from build123d import *

# Parameters (mm, degrees)
SKETCH_1_R                       = 10
EXTRUDE_1_DEPTH                  = 50
SKETCH_2_R                       = 10
EXTRUDE_2_DEPTH                  = 50
SKETCH_3_OUTSIDE_W               = 50.566
SKETCH_3_OUTSIDE_H               = 130.566
SKETCH_3_OUTSIDE_R               = 3
CUT_EXTRUDE_1_DEPTH              = 20
FILLET_2_R                       = 4
PATTERN_CIRCULAR_1_COUNT         = 4
FILLET_2_OF_PATTERN_CIRCULAR_1_R = 4


with BuildPart() as part:
    # Sketch 1 → Extrude 1 (new, symmetric)
    with BuildSketch(Plane(origin=(0, 0, 0), x_dir=(1, 0, 0), z_dir=(0, 1, 0))):
        with Locations(Location((0, 0, 0), (0, 0, 90))):
            Circle(SKETCH_1_R)
    extrude(amount=EXTRUDE_1_DEPTH, both=True)

    # Sketch 2 → Extrude 2 (add, symmetric)
    with BuildSketch(Plane(origin=(0, 0, 0), x_dir=(0, 0, -1), z_dir=(1, 0, 0))):
        Circle(SKETCH_2_R)
    extrude(amount=EXTRUDE_2_DEPTH, both=True)

    # Sketch 3 outside → Cut-Extrude 1 (cut)
    with BuildSketch(Plane.ZY.offset(50)):
        Rectangle(SKETCH_3_OUTSIDE_W, SKETCH_3_OUTSIDE_H)
        Circle(SKETCH_3_OUTSIDE_R, mode=Mode.SUBTRACT)
    cut_extrude_1 = extrude(amount=-CUT_EXTRUDE_1_DEPTH, mode=Mode.SUBTRACT)

    # Fillet 2
    fillet_2_edges = [part.edges().sort_by_distance(p)[0] for p in [
        (-30, 0, -3),
    ]]
    fillet(fillet_2_edges, radius=FILLET_2_R)

    # Pattern Circular 1: Cut-Extrude 1 ×4 about axis
    pattern_circular_1_axis = Axis((0, 0, 0), (0, 0, 1))
    for i in range(1, PATTERN_CIRCULAR_1_COUNT):
        add(cut_extrude_1.rotate(pattern_circular_1_axis, i * 360 / PATTERN_CIRCULAR_1_COUNT), mode=Mode.SUBTRACT)

    # Fillet 2 of Pattern Circular 1
    fillet_2_of_pattern_circular_1_edges = [part.edges().sort_by_distance(p)[0] for p in [
        (0, -30, -3),
        (30, 0, -3),
        (0, 30, -3),
    ]]
    fillet(fillet_2_of_pattern_circular_1_edges, radius=FILLET_2_OF_PATTERN_CIRCULAR_1_R)


solid = part.part
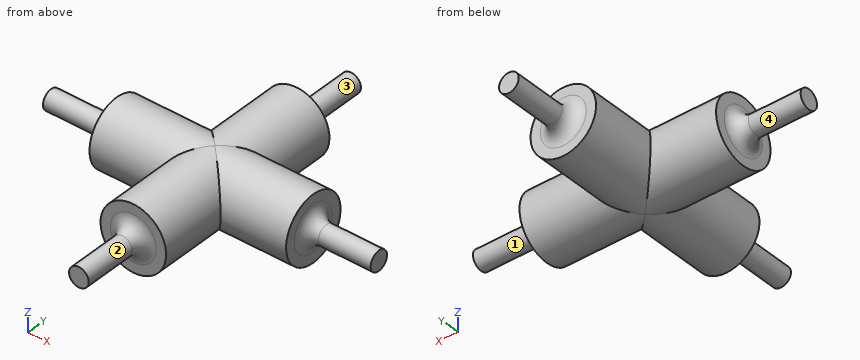
Input: part model. Units: mm. Frame: model coordinates. Face numbers are marked on the shaded views. A direction names the side the tool comes from. Coordinates: 2 decimals unless noted, no trailing zeros. Order: outer loops, then holes, each group sorted by start corner. A loop starts at its lowest first (then second) coordinate and runs counter-clockwise, first axis right, second up. Notation, with made-up numbers: M 16,8.5 L 27,8.5 A15 ccw 27,26.5 Z; hole C -7.75,3 d3. An arc over 180 degrees is marked long. One line per question, with ' | ' between items.
Item 1: Section B-B (x = -26). Output: boundary loops of the cut face in (y, z), then the cut area to 3 significant figures.
Geometry results:
outline: C 0,0 d20 | area: 314 mm^2
Item 2: Ray query, line 1 along Y through (x, z) = (8.5, -0.25); line 2 along X through (y, z) = (15, 0.25); line 3 along Y through (x, z) = (41.5, -1). Return the intervals inside material, ascending.
Geometry results:
line 1: y = -30 to 30 | line 2: x = -10 to 10 | line 3: y = -2.83 to 2.83
Item 3: Pin query (flat end, axial travel): pin 1 (8 mm diameter, centred on y = -16, z = -6.5, fed in from -X); pin 2 (2 mm diameter, centred on x = -19.5, z = -6.5, fed in from +Y); pin 3 (6 mm diameter, centred on x = 27.5, z = 8, fed in from +Y); pin 4 (6 mm diameter, centred on y = -3.5, z = -1, fed in from +X). Return the tip coordinate at first contact, or that it passes through.
Geometry results:
pin 1: stops at x = -9.68 | pin 2: stops at y = 8.35 | pin 3: stops at y = 8.66 | pin 4: stops at x = 50
Item 4: Reachability of the marked faces 1, 2, 3 and 4 from +Z, -Z, +X, -X, +Y, -Y: full face, straight path, thin tool, end or side. Return the list, or none.
Geometry results:
face 1: +X | face 2: -Y | face 3: +Y | face 4: -X
Item 5: Section A-A (z = -8.25). Output: boundary loops of the cut face in (x, y).
Geometry results:
outline: M -30,-5.65 L -5.65,-5.65 L -5.65,-30 L 5.65,-30 L 5.65,-5.65 L 30,-5.65 L 30,5.65 L 5.65,5.65 L 5.65,30 L -5.65,30 L -5.65,5.65 L -30,5.65 Z
